from build123d import *

# Parameters (mm, degrees)
EXTRUDE_1_DEPTH      = 17.5
EXTRUDE_1_DEPTH_BACK = 17.5
SKETCH_2_W           = 35
SKETCH_2_H           = 28
CUT_EXTRUDE_1_DEPTH  = 35
CUT_EXTRUDE_2_DEPTH  = 6
CUT_EXTRUDE_3_DEPTH  = 6
SKETCH_5_W           = 9
SKETCH_5_H           = 28
SKETCH_5_W_2         = 5.8
SKETCH_5_H_2         = 35
CUT_EXTRUDE_4_DEPTH  = 3.2
SKETCH_6_W           = 28
SKETCH_6_H           = 9
SKETCH_6_W_2         = 35
SKETCH_6_H_2         = 6
CUT_EXTRUDE_5_DEPTH  = 3.2
SKETCH_8_W           = 2
SKETCH_8_H           = 2
EXTRUDE_2_DEPTH      = 3.9
EXTRUDE_2_DEPTH_BACK = 3.9
FILLET_2_R           = 0.5


with BuildPart() as part:
    # Sketch 1 → Extrude 1 (new body, two sides)
    with BuildSketch(Plane.XY) as extrude_1_sk:
        Polygon((0, 0), (0, 40), (7.8, 40), (7.8, 32.2), (32.2, 7.8), (40, 7.8), (40, 0), align=None)
    extrude(amount=EXTRUDE_1_DEPTH)
    extrude(extrude_1_sk.sketch, amount=-EXTRUDE_1_DEPTH_BACK)

    # Sketch 2 → Cut-Extrude 1 (cut)
    with BuildSketch(Plane(origin=(0, 40, 0), x_dir=(1, 0, 0), z_dir=(0, 1, 0))):
        with Locations((22.5, 0)):
            Rectangle(SKETCH_2_W, SKETCH_2_H)
    extrude(amount=-CUT_EXTRUDE_1_DEPTH, mode=Mode.SUBTRACT)

    # Sketch 3 → Cut-Extrude 2 (cut, through all)
    with BuildSketch(Plane(origin=(0, 5, 0), x_dir=(1, 0, 0), z_dir=(0, 1, 0))):
        with BuildLine():
            Line((14, 4.5), (27, 4.5))
            ThreePointArc((27, 4.5), (31.5, 0), (27, -4.5))
            Line((27, -4.5), (14, -4.5))
            ThreePointArc((14, -4.5), (9.5, 0), (14, 4.5))
        make_face()
    extrude(amount=-CUT_EXTRUDE_2_DEPTH, mode=Mode.SUBTRACT)

    # Sketch 4 → Cut-Extrude 3 (cut, through all)
    with BuildSketch(Plane(origin=(5, 0, 0), x_dir=(0, 0, -1), z_dir=(1, 0, 0))):
        with BuildLine():
            Line((4.5, 27), (4.5, 14))
            ThreePointArc((4.5, 14), (0, 9.5), (-4.5, 14))
            Line((-4.5, 14), (-4.5, 27))
            ThreePointArc((-4.5, 27), (0, 31.5), (4.5, 27))
        make_face()
    extrude(amount=-CUT_EXTRUDE_3_DEPTH, mode=Mode.SUBTRACT)

    # Sketch 5 → Cut-Extrude 4 (cut)
    with BuildSketch(Plane.ZY):
        with Locations((0, 20)):
            Rectangle(SKETCH_5_W, SKETCH_5_H)
        with Locations((-11.6, 19.5)):
            Rectangle(SKETCH_5_W_2, SKETCH_5_H_2)
        with Locations((11.6, 19.5)):
            Rectangle(SKETCH_5_W_2, SKETCH_5_H_2)
    extrude(amount=-CUT_EXTRUDE_4_DEPTH, mode=Mode.SUBTRACT)

    # Sketch 6 → Cut-Extrude 5 (cut)
    with BuildSketch(Plane.XZ):
        with Locations((20, 0)):
            Rectangle(SKETCH_6_W, SKETCH_6_H)
        with Locations((20.5, 11)):
            Rectangle(SKETCH_6_W_2, SKETCH_6_H_2)
        with Locations((20.5, -11)):
            Rectangle(SKETCH_6_W_2, SKETCH_6_H_2)
    extrude(amount=-CUT_EXTRUDE_5_DEPTH, mode=Mode.SUBTRACT)

    # Sketch 8 → Extrude 2 (add, two sides)
    with BuildSketch(Plane.XY) as extrude_2_sk:
        with Locations((-1, 35)):
            Rectangle(SKETCH_8_W, SKETCH_8_H)
        with Locations((-1, 5)):
            Rectangle(SKETCH_8_W, SKETCH_8_H)
        with Locations((5, -1)):
            Rectangle(SKETCH_8_W, SKETCH_8_H)
        with Locations((35, -1)):
            Rectangle(SKETCH_8_W, SKETCH_8_H)
    extrude(amount=EXTRUDE_2_DEPTH)
    extrude(extrude_2_sk.sketch, amount=-EXTRUDE_2_DEPTH_BACK)

    # Fillet 2
    fillet_2_edges = [part.edges().sort_by_distance(p)[0] for p in [
        (-1, 34, -3.9),
        (-1, 36, -3.9),
        (-1, 36, 3.9),
        (-1, 34, 3.9),
        (-1, 6, -3.9),
        (-1, 4, -3.9),
        (-1, 6, 3.9),
        (-1, 4, 3.9),
        (6, -1, -3.9),
        (4, -1, -3.9),
        (4, -1, 3.9),
        (6, -1, 3.9),
        (36, -1, -3.9),
        (34, -1, -3.9),
        (34, -1, 3.9),
        (36, -1, 3.9),
    ]]
    fillet(fillet_2_edges, radius=FILLET_2_R)


solid = part.part
Geometry check sheet. Reference: the model listing, model coordinates, mm. A direction names the side the tool comes from. Round coordinates to 2 decimals unless told otherwise and drop trailing zeros. Order: outer loops, then holes, each group sorted by start corner. A loop starts at its lowest first (then second) coordinate and runs counter-clockwise, first axis right, second up. Notation, with made-up numbers: M 42.5,57.25 L 70.5,57.25 A34 cw 70.5,89.25 Z; hole C 27,76 d5. An arc over 180 degrees is marked long. Answer in a Markdown table with one row per item.
(1) Sectioned sample at B-B, the plane z = 0. State how many separate pieces and enclosed holes the cut face has, and give its area (3 significant figures).
Responses:
| item | result |
|---|---|
| separate pieces | 3 |
| enclosed holes | 0 |
| area | 133 mm² |
(2) Go/stop test with flat-tipped pins: P1, Ø10, axis at x = 17, z = -4, coming from the +Y side; P2, Ø3.5, axis at x = 31.5, z = -1, coming from the -Y side; P3, Ø1.1, axis at x = -1.5, y = 35, coming from the +Z side. Record where each tip stops, or that it passes through.
Responses:
| item | result |
|---|---|
| P1 | stops at y = 5 |
| P2 | stops at y = 3.2 |
| P3 | stops at z = 3.9 |
(3) Sectioned sample at A-A, the plane x = 24. Record the cut outline in (y, z).
Responses:
| item | result |
|---|---|
| outline | M 0,-17.5 L 16,-17.5 L 16,-14 L 5,-14 L 5,-4.5 L 0,-4.5 L 0,-8 L 3.2,-8 L 3.2,-14 L 0,-14 Z; M 0,4.5 L 5,4.5 L 5,14 L 16,14 L 16,17.5 L 0,17.5 L 0,14 L 3.2,14 L 3.2,8 L 0,8 Z |
(4) Draft check along X on faces 4 (the face through (38, 2, -11)), 5 (the face through (20.3, 0, -7.5)), 6 (the face through (3.2, 8, 0)). Enter one of: released by +X, released by -X, zero draft, split by the parting line, or undercut.
Responses:
| item | result |
|---|---|
| face 4 | undercut |
| face 5 | zero draft |
| face 6 | released by -X |
(5) Tool access check on faces 1 (the face through (-1, 36, 0)), 2 (the face through (9.5, 4.1, 0.1)), 3 (the face through (20, 2, 8)). Record the directions out of +Z, -Z, +X, -X, +Y, -Y that give a thin tool (end or side, any length) a straight path to the whole face; none if there is none.
Responses:
| item | result |
|---|---|
| face 1 | +Z, -Z, -X, +Y |
| face 2 | +Y, -Y |
| face 3 | -Y |
(6) Sectioned sample at C-C, the plane x = 16.5. Record the cut outline in (y, z), and give its area (3 significant figures).
Responses:
| item | result |
|---|---|
| outline | M 0,-17.5 L 23.5,-17.5 L 23.5,-14 L 5,-14 L 5,-4.5 L 0,-4.5 L 0,-8 L 3.2,-8 L 3.2,-14 L 0,-14 Z; M 0,4.5 L 5,4.5 L 5,14 L 23.5,14 L 23.5,17.5 L 0,17.5 L 0,14 L 3.2,14 L 3.2,8 L 0,8 Z |
| area | 221 mm² |
(7) Scan lines: probe 1 along Z at (x, y) = (1.5, 28.5); probe 2 along Z at (x, y) = (17.5, 20.5); probe 3 along Z at (x, y) = (23, 4). Record each from-to range of solid material in increasing order. Write a range as from..to.
Responses:
| item | result |
|---|---|
| probe 1 | z = -17.5..-14.5, -8.7..-4.5, 4.5..8.7, 14.5..17.5 |
| probe 2 | z = -17.5..-14, 14..17.5 |
| probe 3 | z = -17.5..-4.5, 4.5..17.5 |
